Read the model definition and answer for the solid it produces. Units are mm, in the model's axes. Give positions to 0.01 mm unless a question says otherwise; leave off trailing zeros. Loops run counter-clockwise (first coordinate to the right, second up) from the corner with the lowest first, then second, coordinate; pieces in that order, holes last.
(1) Find section C-C, the plane z = 3.05. Write down the section's boundary in (x, y), then the cut area to 3 significant figures.
(2) Straight lines are drawn through the part: probe 1 along Z at (x, y) = (-40.5, 10.5); probe 2 along Y at (x, z) = (-67.8, 1.35); probe 3 along Y at (x, z) = (-32.8, 0.85). For each, find the intervals that lie inside material, in ascending order.
(3) Find section B-B, the plane y = -7.87. Write down the section's boundary in (x, z), then the cut area to 3 significant figures.
(4) Find section A-A, the plane x = 22.2. Write down the section's boundary in (y, z), then the cut area to 3 significant figures.
(5) Find section D-D, the plane x = 58.77. Write down the section's boundary in (y, z).
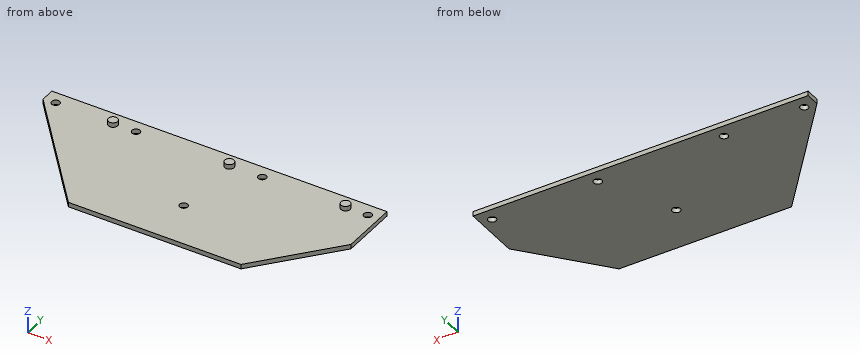
```python
from build123d import *

# Parameters (mm, degrees)
RESSALTO_EXTRUS_O1_DEPTH = 2
CORTE_EXTRUS_O1_REACH    = 4
ESBO_O2_R                = 1.75
ESBO_O3_R                = 2
RESSALTO_EXTRUS_O2_DEPTH = 2


with BuildPart() as part:
    # Esboço1 → Ressalto-extrusão1 (new body)
    with BuildSketch(Plane.XY):
        Polygon((-73, 22.58983114), (-29.645188864, -28.75), (45.554811136, -28.75), (73, 3.75), (73, 28.75), (-73, 28.75), align=None)
    extrude(amount=RESSALTO_EXTRUS_O1_DEPTH)

    # Esboço2 → Corte-extrusão1 (cut, up to next)
    with BuildSketch(Plane.XY.offset(2), mode=Mode.PRIVATE) as corte_extrus_o1_sk1:
        with Locations((22.2, 23.13)):
            Circle(ESBO_O2_R)
    corte_extrus_o1_tool1 = extrude(corte_extrus_o1_sk1.sketch, amount=-CORTE_EXTRUS_O1_REACH, mode=Mode.PRIVATE) & part.part
    add(corte_extrus_o1_tool1.solids().sort_by_distance((22.2, 23.13, 2))[0], mode=Mode.SUBTRACT)
    # Esboço2 → Corte-extrusão1 (cut, up to next)
    with BuildSketch(Plane.XY.offset(2), mode=Mode.PRIVATE) as corte_extrus_o1_sk2:
        with Locations((68.2, 23.13)):
            Circle(ESBO_O2_R)
    corte_extrus_o1_tool2 = extrude(corte_extrus_o1_sk2.sketch, amount=-CORTE_EXTRUS_O1_REACH, mode=Mode.PRIVATE) & part.part
    add(corte_extrus_o1_tool2.solids().sort_by_distance((68.2, 23.13, 2))[0], mode=Mode.SUBTRACT)
    # Esboço2 → Corte-extrusão1 (cut, up to next)
    with BuildSketch(Plane.XY.offset(2), mode=Mode.PRIVATE) as corte_extrus_o1_sk3:
        with Locations((-32.8, 23.13)):
            Circle(ESBO_O2_R)
    corte_extrus_o1_tool3 = extrude(corte_extrus_o1_sk3.sketch, amount=-CORTE_EXTRUS_O1_REACH, mode=Mode.PRIVATE) & part.part
    add(corte_extrus_o1_tool3.solids().sort_by_distance((-32.8, 23.13, 2))[0], mode=Mode.SUBTRACT)
    # Esboço2 → Corte-extrusão1 (cut, up to next)
    with BuildSketch(Plane.XY.offset(2), mode=Mode.PRIVATE) as corte_extrus_o1_sk4:
        with Locations((-67.8, 23.13)):
            Circle(ESBO_O2_R)
    corte_extrus_o1_tool4 = extrude(corte_extrus_o1_sk4.sketch, amount=-CORTE_EXTRUS_O1_REACH, mode=Mode.PRIVATE) & part.part
    add(corte_extrus_o1_tool4.solids().sort_by_distance((-67.8, 23.13, 2))[0], mode=Mode.SUBTRACT)
    # Esboço2 → Corte-extrusão1 (cut, up to next)
    with BuildSketch(Plane.XY.offset(2), mode=Mode.PRIVATE) as corte_extrus_o1_sk5:
        with Locations((7.45, -7.87)):
            Circle(ESBO_O2_R)
    corte_extrus_o1_tool5 = extrude(corte_extrus_o1_sk5.sketch, amount=-CORTE_EXTRUS_O1_REACH, mode=Mode.PRIVATE) & part.part
    add(corte_extrus_o1_tool5.solids().sort_by_distance((7.45, -7.87, 2))[0], mode=Mode.SUBTRACT)

    # Esboço3 → Ressalto-extrusão2 (add)
    with BuildSketch(Plane.XY.offset(2)):
        with Locations((8.17, 22.662028239)):
            Circle(ESBO_O3_R)
        with Locations((58.77, 22.662028239)):
            Circle(ESBO_O3_R)
        with Locations((-42.53, 22.662028239)):
            Circle(ESBO_O3_R)
    extrude(amount=RESSALTO_EXTRUS_O2_DEPTH)


solid = part.part
```
Entries:
1. outline: circle Ø4 at (-42.53, 22.66); circle Ø4 at (8.17, 22.66); circle Ø4 at (58.77, 22.66)
1. area: 37.7 mm2
2. probe 1: z = 0 to 2
2. probe 2: y = 16.43 to 21.38, 24.88 to 28.75
2. probe 3: y = -25.01 to 21.38, 24.88 to 28.75
3. outline: (-47.28, 0) - (5.7, 0) - (5.7, 2) - (-47.28, 2) - close; (9.2, 0) - (63.19, 0) - (63.19, 2) - (9.2, 2) - close
3. area: 214 mm2
4. outline: (-28.75, 0) - (21.38, 0) - (21.38, 2) - (-28.75, 2) - close; (24.88, 0) - (28.75, 0) - (28.75, 2) - (24.88, 2) - close
4. area: 108 mm2
5. outline: (-13.1, 0) - (28.75, 0) - (28.75, 2) - (24.66, 2) - (24.66, 4) - (20.66, 4) - (20.66, 2) - (-13.1, 2) - close
